from build123d import *

# Parameters (mm, degrees)
F1_DEPTH = 25


with BuildPart() as f1:
    # F0 (on Front) → F1 (new body)
    with BuildSketch(Plane.XZ):
        with BuildLine():
            ThreePointArc((-1.457142, 165.198036), (-0.371174, 162.699206), (0, 160))
            Line((0, 160), (0, 0))
            Line((0, 0), (6.307421, 0))
            Line((6.307421, 0), (6.307421, 160))
            ThreePointArc((6.307421, 160), (6.206676, 161.415892), (5.906471, 162.803255))
            ThreePointArc((5.906471, 162.803255), (5.457063, 164.03535), (4.850279, 165.198036))
            Line((4.850279, 165.198036), (-16.398177, 200.119405))
            Line((-16.398177, 200.119405), (-22.632944, 200))
            Line((-22.632944, 200), (-1.457142, 165.198036))
        make_face()
    extrude(amount=F1_DEPTH)


solid = f1.part
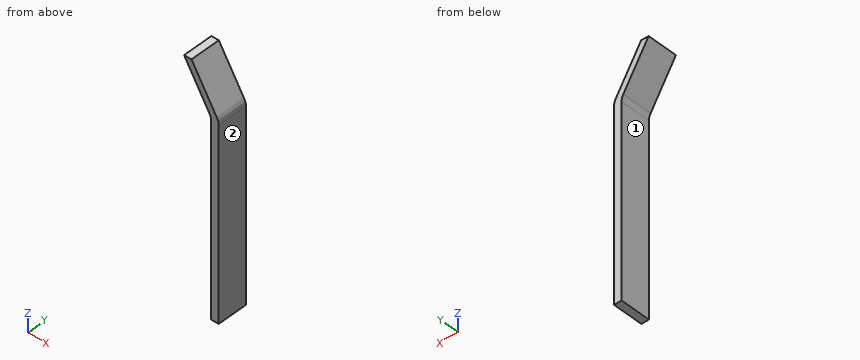
Model file for the job. Use its own axes, mm. Face numbers are marked on the shaded views. A direction names the side the tool comes from. Give positions to 0.01 mm unless a question says otherwise; leave off trailing zeros. Order: outer loops, then holes, each group sorted by start corner. A loop starts at its lowest first (then second) coordinate and runs counter-clockwise, first axis right, second up. Notation, with made-up numbers: (-16.75, 74.5) - (37.25, 74.5) arc R27 cw to (37.25, 108.5) - close; hole circle Ø6 at (52, 12). An arc over 180 degrees is marked (long way). Write item = value, one per line. Start each with the question number.
1. Drop flat-ended pins along their axis: P1, Ø2, axis at x = 3, y = -20.5, coming from the -Z side; P2, Ø5, axis at y = -13, z = 53, coming from the -X side; P3, Ø6, axis at x = 1, y = -20, coming from the +Z side; P4, Ø12, axis at x = 3, y = -21, coming from the +Z side. Give the stop position or say it passes through.
2. Cut at B-B, the plane z = 57. List the corners of the cut face in (x, y).
3. Cut at A-A, the plane y = -5.25. List the corners of the cut face in (x, z), and give its area (3 significant figures).
4. Which spindle directions (+Z, -Z, +X, -X, +Y, -Y) get a long thin tool onto all of the face, cutting with end or side? Do the marked faces 1 and 2. Say none if no direction does.
5. Cut at C-C, the plane x = 3. List the corners of the cut face in (y, z), and give its area (3 significant figures).
6. Probe line 1 along X through (y, z) = (-10.5, 46.5); line 2 along Z through (x, y) = (-18.5, -12.75); line 3 along Z through (x, y) = (-1.25, -9). List the from-to ranges inside material, lowest first.
Taken from the geometry:
q1.P1 = 0
q1.P2 = 0
q1.P3 = 176.46
q1.P4 = 178.1
q2.outline = (0, -25) - (6.31, -25) - (6.31, 0) - (0, 0) - close
q3.outline = (-22.63, 200) - (-1.46, 165.2) arc R10 cw to (0, 160) - (0, 0) - (6.31, 0) - (6.31, 160) arc R10 ccw to (5.91, 162.8) arc R10 ccw to (4.85, 165.2) - (-16.4, 200.12) - close
q3.area = 1,260 mm²
q4.face_1 = -Z, -X, +Y, -Y
q4.face_2 = +Z, -Z, +X, +Y, -Y
q5.outline = (-25, 0) - (0, 0) - (0, 168.24) - (-25, 168.24) - close
q5.area = 4,210 mm²
q6.line_1 = 0 to 6.31
q6.line_2 = 193.21 to 200.08
q6.line_3 = 164.84 to 175.22
